Geometry: final body of the model. Coordinates: model frame, mm. Round coordinates to 2 decimals unless told otherwise and drop trailing zeros. Loops run counter-clockwise (first coordinate to the right, second up) from the corner with the lowest first, then second, coordinate; pieces in that order, holes last. Notation, with made-up numbers: M 15,9 L 69,9 A22 cw 69,46 Z; hole C 18.5,42 d9. An arc over 180 degrees is marked long. Return JSON: item names as keys, results as strings.
from build123d import *

# Parameters (mm, degrees)
SKETCH_1_R      = 1.5
SKETCH_1_R_2    = 1
EXTRUDE_1_DEPTH = 2


with BuildPart() as part:
    # 草图1 → 凸台-拉伸1 (new body)
    with BuildSketch(Plane.XY):
        with BuildLine():
            ThreePointArc((8.708571429, 121.645714286), (-0.291428571, 130.645714286), (-9.291428571, 121.645714286))
            Line((-9.291428571, 121.645714286), (-9.291428571, 21.645714286))
            Line((-9.291428571, 21.645714286), (-33.291428571, 21.645714286))
            Line((-33.291428571, 21.645714286), (-60.986481548, -7.354285714))
            Line((-60.986481548, -7.354285714), (-60.986481548, -15.354285714))
            Line((-60.986481548, -15.354285714), (60.403624405, -15.354285714))
            Line((60.403624405, -15.354285714), (60.403624405, -7.354285714))
            Line((60.403624405, -7.354285714), (32.708571429, 21.645714286))
            Line((32.708571429, 21.645714286), (8.708571429, 21.645714286))
            Line((8.708571429, 21.645714286), (8.708571429, 121.645714286))
        make_face()
        with Locations((-49.791428571, -7.354285714)):
            Circle(SKETCH_1_R, mode=Mode.SUBTRACT)
        with Locations((-33.291428571, 7.645714286)):
            Circle(SKETCH_1_R, mode=Mode.SUBTRACT)
        with Locations((-0.291428571, 37.645714286)):
            Circle(SKETCH_1_R, mode=Mode.SUBTRACT)
        with Locations((49.208571429, -7.354285714)):
            Circle(SKETCH_1_R, mode=Mode.SUBTRACT)
        with Locations((32.708571429, 7.645714286)):
            Circle(SKETCH_1_R, mode=Mode.SUBTRACT)
        with Locations((-6.291428571, 121.645714286)):
            Circle(SKETCH_1_R_2, mode=Mode.SUBTRACT)
        with Locations((5.708571429, 121.645714286)):
            Circle(SKETCH_1_R_2, mode=Mode.SUBTRACT)
    extrude(amount=EXTRUDE_1_DEPTH)


solid = part.part
Q1. Section query B-B (x = -13). Output: boundary loops of the cut face in (y, z), plus the area to 3 significant figures.
Determined:
{"outline": "M -15.35,0 L 21.65,0 L 21.65,2 L -15.35,2 Z", "area": "74.0 mm^2"}
Q2. Section query A-A (z = 0.8). Output: boundary loops of the cut face in (x, y).
Determined:
{"outline": "M -60.99,-15.35 L 60.4,-15.35 L 60.4,-7.35 L 32.71,21.65 L 8.71,21.65 L 8.71,121.65 A9 ccw -9.29,121.65 L -9.29,21.65 L -33.29,21.65 L -60.99,-7.35 Z; hole C -49.79,-7.35 d3; hole C -33.29,7.65 d3; hole C -6.29,121.65 d2; hole C -0.29,37.65 d3; hole C 5.71,121.65 d2; hole C 32.71,7.65 d3; hole C 49.21,-7.35 d3"}
Q3. Material intervals for L1, parallel to Y at x = 11, z = 1.85; L2, parallel to Y at x = 34, z = 1.75; L3, parallel to X at y = 114.5, z = 0.25, sorted ascending.
Determined:
{"L1": "y = -15.35 to 21.65", "L2": "y = -15.35 to 6.88, 8.41 to 20.29", "L3": "x = -9.29 to 8.71"}
Q4. Pull-direction query (Y, two-part tool) for faces 1 (the flat face through (-46.945, 7.349, 0.986)), 2 (the flat face through (-1, 31, 0)), 3 (the cylindrical face through (34.094, 7.071, 0.986)); classes: pulls with the +Y half, pulls with the -Y half, needs draft (parallel to the pull), parting line crosses it, or undercut.
Determined:
{"face 1": "pulls with the +Y half", "face 2": "needs draft", "face 3": "undercut"}
Q5. Section query C-C (y = 49). Output: boundary loops of the cut face in (x, z), plus the area to 3 significant figures.
Determined:
{"outline": "M -9.29,0 L 8.71,0 L 8.71,2 L -9.29,2 Z", "area": "36.0 mm^2"}
Q6. Pin query (flat end, axial travel): pin 1 (1.6 mm diameter, centred on x = 5.71, y = 121.65, fed in from -Z); pin 2 (1 mm diameter, centred on x = 20.5, z = 1.5, fed in from +Y); pin 3 (4 mm diameter, centred on x = -33.29, y = 7.65, fed in from +Z); pin 4 (1 mm diameter, centred on y = 23.5, z = 1.5, fed in from +X). Return the tip coordinate at first contact, or that it passes through.
Determined:
{"pin 1": "passes through", "pin 2": "stops at y = 21.65", "pin 3": "stops at z = 2", "pin 4": "stops at x = 8.71"}
